Design review of the part built by this model. Coordinates are the model's own, in mm. Face numbers are marked on the shaded views. A direction names the side the tool comes from. Give positions to 0.01 mm unless a question says otherwise; leave off trailing zeros. Order: outer loops, then holes, each group sorted by start corner. A loop starts at its lowest first (then second) coordinate and runs counter-clockwise, first axis right, second up. Notation, with made-up numbers: (81.5, 16.25) -> (109.5, 16.25) arc R8 ccw to (109.5, 30.25) -> close; hole circle Ø5 at (22, -23.5). An arc over 180 degrees is marked (long way). Return JSON: item names as keys, results as strings.
```python
from build123d import *

# Parameters (mm, degrees)
SZKIC1_R                    = 10
DODANIE_WYCI_GNI_CIE1_DEPTH = 10
SZKIC2_W                    = 10
SZKIC2_H                    = 120
DODANIE_WYCI_GNI_CIE2_DEPTH = 65
ZAOKR_GLENIE1_R             = 10
SZKIC4_R                    = 12.5
WYTNIJ_WYCI_GNI_CIE1_DEPTH  = 65


with BuildPart() as part:
    # Szkic1 → Dodanie-wyciągnięcie1 (new body)
    with BuildSketch(Plane.XY):
        with BuildLine():
            Line((-130, 87.5), (130, 87.5))
            ThreePointArc((130, 87.5), (144.142135624, 81.642135624), (150, 67.5))
            Line((150, 67.5), (150, -67.5))
            ThreePointArc((150, -67.5), (144.142135624, -81.642135624), (130, -87.5))
            Line((130, -87.5), (-130, -87.5))
            ThreePointArc((-130, -87.5), (-144.142135624, -81.642135624), (-150, -67.5))
            Line((-150, -67.5), (-150, 67.5))
            ThreePointArc((-150, 67.5), (-144.142135624, 81.642135624), (-130, 87.5))
        make_face()
        with Locations((-130, 67.5)):
            Circle(SZKIC1_R, mode=Mode.SUBTRACT)
        with Locations((-130, -67.5)):
            Circle(SZKIC1_R, mode=Mode.SUBTRACT)
        with Locations((130, -67.5)):
            Circle(SZKIC1_R, mode=Mode.SUBTRACT)
        with Locations((130, 67.5)):
            Circle(SZKIC1_R, mode=Mode.SUBTRACT)
    extrude(amount=DODANIE_WYCI_GNI_CIE1_DEPTH)

    # Szkic2 → Dodanie-wyciągnięcie2 (add)
    with BuildSketch(Plane.XY.offset(10)):
        Rectangle(SZKIC2_W, SZKIC2_H)
    extrude(amount=DODANIE_WYCI_GNI_CIE2_DEPTH)

    # Zaokrąglenie1
    zaokr_glenie1_edges = [part.edges().sort_by_distance(p)[0] for p in [
        (0, 60, 75),
        (0, -60, 75),
    ]]
    fillet(zaokr_glenie1_edges, radius=ZAOKR_GLENIE1_R)

    # Szkic4 → Wytnij-wyciągnięcie1 (cut)
    with BuildSketch(Plane(origin=(5, 0, 0), x_dir=(0, 0, -1), z_dir=(1, 0, 0))):
        with Locations(Location((-55, 0, 0), (0, 0, 90))):
            Circle(SZKIC4_R)
    extrude(amount=-WYTNIJ_WYCI_GNI_CIE1_DEPTH, mode=Mode.SUBTRACT)


solid = part.part
```
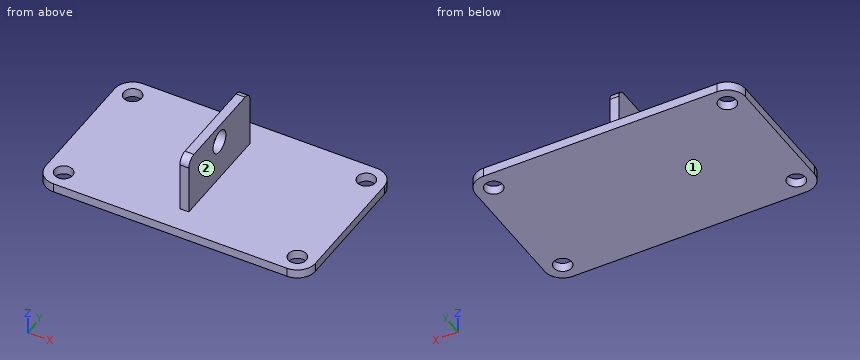
Item 1: Add section C-C (y = 44.5). Give the boundary of the cut face in (x, z).
Result set:
{"outline": "(-150, 0) -> (150, 0) -> (150, 10) -> (5, 10) -> (5, 75) -> (-5, 75) -> (-5, 10) -> (-150, 10) -> close"}
Item 2: Add section D-D (x = -26.5). Give the boundary of the cut face in (y, z), plus the area to 3 significant figures.
Result set:
{"outline": "(-87.5, 0) -> (87.5, 0) -> (87.5, 10) -> (-87.5, 10) -> close", "area": "1,750 mm^2"}
Item 3: Wall thickness on L1, parallel to Y at x = -130, z = 6.5; L2, parallel to X at y = 67, z = 5; L3, parallel to Z at x = 0.25, y = 0: over which ranges is each line inside the solid? List them lowest first. Write a range as [from, to].
Result set:
{"L1": "y = [-87.5, -77.5], [-57.5, 57.5], [77.5, 87.5]", "L2": "x = [-150, -139.99], [-120.01, 120.01], [139.99, 150]", "L3": "z = [0, 42.5], [67.5, 75]"}
Item 4: Machinability: for the marked faces 1 and 2, which of the approach directions +Z, -Z, +X, -X, +Y, -Y give a long, thin tool a straight path to every point of the face, cutting with its end or side? Answer none if there is none.
Result set:
{"face 1": "-Z, +X, -X, +Y, -Y", "face 2": "+Z, +X, +Y, -Y"}
Item 5: Add section A-A (y = 0). Give the boundary of the cut face in (x, z).
Result set:
{"outline": "(-150, 0) -> (150, 0) -> (150, 10) -> (5, 10) -> (5, 42.5) -> (-5, 42.5) -> (-5, 10) -> (-150, 10) -> close; (-5, 67.5) -> (5, 67.5) -> (5, 75) -> (-5, 75) -> close"}
Item 6: For pin 1 (8 mm diameter, centred on x = 1, z = 38.5, fed in from -Y); pin 2 (12 mm diameter, centred on y = -54.5, z = 66.5, fed in from +X); pin 3 (3 mm diameter, centred on x = -2, z = 38.5, fed in from +Y), all flat-tipped, find the tip position at first contact; note any pin that passes through.
Result set:
{"pin 1": "stops at y = -60", "pin 2": "stops at x = 5", "pin 3": "stops at y = 60"}
Item 7: Add section B-B (z = 55). Give the boundary of the cut face in (x, y), plus the area to 3 significant figures.
Result set:
{"outline": "(-5, -60) -> (5, -60) -> (5, -12.5) -> (-5, -12.5) -> close; (-5, 12.5) -> (5, 12.5) -> (5, 60) -> (-5, 60) -> close", "area": "950 mm^2"}
